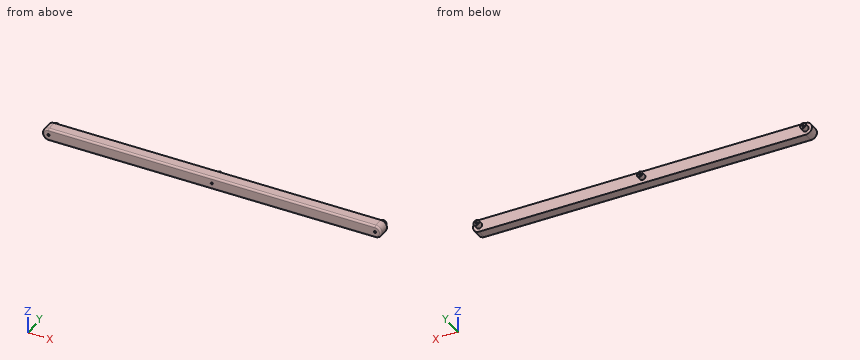
```python
from build123d import *

# Parameters (mm, degrees)
SALIENTE_EXTRUIR1_DEPTH = 3
CROQUIS3_R              = 1.59
SALIENTE_EXTRUIR2_DEPTH = 3
REDONDEO1_R             = 1
CROQUIS4_R              = 0.59
CORTAR_EXTRUIR1_DEPTH   = 94.945755625


with BuildPart() as part:
    # Croquis2 → Saliente-Extruir1 (new, symmetric)
    with BuildSketch(Plane(origin=(0, 0, 0), x_dir=(1, 0, 0), z_dir=(0, 1, 0))):
        with BuildLine():
            Line((-90, -3.45), (90, -3.45))
            ThreePointArc((90, -3.45), (93.45, 0), (90, 3.45))
            Line((90, 3.45), (-90, 3.45))
            ThreePointArc((-90, 3.45), (-93.45, 0), (-90, -3.45))
        make_face()
    extrude(amount=SALIENTE_EXTRUIR1_DEPTH, both=True)

    # Croquis3 → Saliente-Extruir2 (add)
    with BuildSketch(Plane(origin=(0, 3, 0), x_dir=(1, 0, 0), z_dir=(0, 1, 0))):
        with Locations(Location((-90, 0, 0), (0, 0, 270))):
            Circle(CROQUIS3_R)
        with Locations(Location((90, 0, 0), (0, 0, 270))):
            Circle(CROQUIS3_R)
        with Locations(Location((0, 0, 0), (0, 0, 270))):
            Circle(CROQUIS3_R)
    extrude(amount=SALIENTE_EXTRUIR2_DEPTH)

    # Redondeo1
    redondeo1_edges = [part.edges().sort_by_distance(p)[0] for p in [
        (0, -3, -3.45),
        (93.45, -3, 0),
        (0, -3, 3.45),
        (-93.45, -3, 0),
    ]]
    fillet(redondeo1_edges, radius=REDONDEO1_R)

    # Croquis4 → Cortar-Extruir1 (cut, through all)
    with BuildSketch(Plane(origin=(0, 6, 0), x_dir=(1, 0, 0), z_dir=(0, 1, 0))):
        with Locations(Location((90, 0, 0), (0, 0, 270))):
            Circle(CROQUIS4_R)
        with Locations(Location((-90, 0, 0), (0, 0, 270))):
            Circle(CROQUIS4_R)
        with Locations(Location((0, 0, 0), (0, 0, 270))):
            Circle(CROQUIS4_R)
    extrude(amount=-CORTAR_EXTRUIR1_DEPTH, mode=Mode.SUBTRACT)


solid = part.part
```
Work out the finished part from the listing and answer in its coordinate system (mm). Coordinates: 2 decimals unless noted, no trailing zeros. Loops run counter-clockwise (first coordinate to the right, second up) from the corner with the lowest first, then second, coordinate; pieces in that order, holes last.
1) Section A-A (y = 4.5) is taken. Give the vertices of the cut face in (x, z), plus the area to 3 significant figures.
Results:
outline: circle Ø3.18 at (-90, 0); circle Ø3.18 at (0, 0); circle Ø3.18 at (90, 0); hole circle Ø1.18 at (-90, 0); hole circle Ø1.18 at (0, 0); hole circle Ø1.18 at (90, 0)
area: 20.5 mm2
2) Consider probe 1 along X at (y, z) = (2, 0); probe 2 along X at (y, z) = (3.25, 0); probe 3 along X at (y, z) = (-1, -0.5). Determine where each line is inside the solid, lowest interval first.
Results:
probe 1: x = -93.45 to -90.59, -89.41 to -0.59, 0.59 to 89.41, 90.59 to 93.45
probe 2: x = -91.59 to -90.59, -89.41 to -88.41, -1.59 to -0.59, 0.59 to 1.59, 88.41 to 89.41, 90.59 to 91.59
probe 3: x = -93.41 to -90.31, -89.69 to -0.31, 0.31 to 89.69, 90.31 to 93.41
3) A flat-ended cylindrical pin translates along its axis: pin 1 (0.9 mm diameter, centred on x = 90, z = 0, fed in from +Y). Find the tip coordinate at first contact, or state that the pin passes through.
Results:
pin 1: passes through
4) Section B-B (x = 53.5) is taken. Give the vertices of the cut face in (y, z), plus the area to 3 significant figures.
Results:
outline: (-3, -2.45) arc R1 ccw to (-2, -3.45) - (3, -3.45) - (3, 3.45) - (-2, 3.45) arc R1 ccw to (-3, 2.45) - close
area: 41.0 mm2
